Can you work these out from the model? Positions are in its coordinate system, mm. A direction names the side the tool comes from. Coordinates: 2 decimals unless noted, no trailing zeros. Order: outer loops, then holes, each group sorted by start corner. A loop starts at its lowest first (then second) coordinate and runs counter-clockwise, first axis right, second up. Notation, with made-up numbers: (44.25, -5) -> (103.25, -5) arc R30 ccw to (103.25, 19) -> close; hole circle Ø11 at (72.5, -6). An arc over 180 degrees is marked (long way). Answer as a JSON object with one key per item and string values. Group by question number.
(1) I want a section at D-D, the plane x = -5.25. List the corners of the cut face in (y, z) for me (3 decimals).
(2) I want a section at A-A, the plane x = 0. List the corners of the cut face in (y, z) for me (3 decimals).
(3) I want a section at B-B, the plane z = 3. List the corners of the cut face in (x, y) for me.
(4) For pin 1 (2 mm diameter, centred on y = -1, z = 18.5, fed in from +X); pin 2 (4.5 mm diameter, centred on x = -2.5, z = 14.5, fed in from +Y); pin 3 (0.8 mm diameter, centred on y = 0, z = -33, fed in from +X) (3 decimals), each with a flat end and sliding along its axis, tell me the tip position at first contact or that it passes through.
(5) I need wall thicknesses on line 1 (Z direction, x = -8.5, y = -2); line 2 (Y direction, x = -8, z = 7.5); line 3 (Z direction, x = -13, y = -12). Which ranges of each line are inside material? Lowest first, please.
(6) Which directions (+Z, -Z, +X, -X, +Y, -Y) give clear straight access to the entire face, cutting with the end or side of a thin tool? Please do faces 1 (the flat face through (-12, 12, 0)), 2 (the flat face through (9, 0.375, -33)), 3 (the cylindrical face through (15.62, 4.92, -15.16)), 4 (the flat face through (-9, -0.375, -33)), 5 (the cylindrical face through (1.096, -2.107, 31.836)).
(7) I want a section at C-C, the plane y = -8.5. List the corners of the cut face in (x, z) for me, plus the area to 3 significant figures.
from build123d import *

# Parameters (mm, degrees)
PAD_DEPTH    = 27.3
SKETCH001_R  = 16.375
PAD001_DEPTH = 30.75
SKETCH002_R  = 2.375
PAD002_DEPTH = 36.5
SKETCH004_W  = 2
SKETCH004_H  = 0.75
PAD004_DEPTH = 35


with BuildPart() as part:
    # Sketch → Pad (new body)
    with BuildSketch(Plane.XY):
        with BuildLine():
            Line((-16.25, 7.500021), (-16.25, -7.5))
            ThreePointArc((-16.25, -7.5), (-13.687184, -13.687185), (-7.499999, -16.25))
            Line((-7.499999, -16.25), (7.500022, -16.25))
            ThreePointArc((7.500022, -16.25), (13.687191, -13.687191), (16.25, -7.500023))
            Line((16.25, -7.500023), (16.25, 7.499999))
            ThreePointArc((16.25, 7.499999), (13.687185, 13.687184), (7.5, 16.25))
            Line((7.5, 16.25), (-7.500021, 16.25))
            ThreePointArc((-7.500021, 16.25), (-13.687184, 13.687184), (-16.25, 7.500021))
        make_face()
    extrude(amount=PAD_DEPTH)

    # Sketch001 → Pad001 (join)
    with BuildSketch(Plane.XY):
        Circle(SKETCH001_R)
    extrude(amount=-PAD001_DEPTH)

    # Sketch002 → Pad002 (join)
    with BuildSketch(Plane.XY):
        Circle(SKETCH002_R)
        with Locations((-5.25, 12.25)):
            Circle(SKETCH002_R)
    extrude(amount=PAD002_DEPTH)

    # Sketch004 → Pad004 (join)
    with BuildSketch(Plane.XY):
        with Locations((-8.875, 0)):
            Rectangle(SKETCH004_W, SKETCH004_H)
        with Locations((8.875, 0)):
            Rectangle(SKETCH004_W, SKETCH004_H)
    extrude(amount=-PAD004_DEPTH)


solid = part.part
Computed values:
{
 "1": {"outline": "(-16.25, 0) -> (-15.511, 0) -> (-15.511, -30.75) -> (15.511, -30.75) -> (15.511, 0) -> (16.25, 0) -> (16.25, 27.3) -> (14.625, 27.3) -> (14.625, 36.5) -> (9.875, 36.5) -> (9.875, 27.3) -> (-16.25, 27.3) -> close"},
 "2": {"outline": "(-16.375, -30.75) -> (16.375, -30.75) -> (16.375, 0) -> (16.25, 0) -> (16.25, 27.3) -> (2.375, 27.3) -> (2.375, 36.5) -> (-2.375, 36.5) -> (-2.375, 27.3) -> (-16.25, 27.3) -> (-16.25, 0) -> (-16.375, 0) -> close"},
 "3": {"outline": "(-16.25, -7.5) arc R8.75 ccw to (-7.5, -16.25) -> (7.5, -16.25) arc R8.75 ccw to (16.25, -7.5) -> (16.25, 7.5) arc R8.75 ccw to (7.5, 16.25) -> (-7.5, 16.25) arc R8.75 ccw to (-16.25, 7.5) -> close"},
 "4": {"pin 1": "stops at x = 16.25", "pin 2": "stops at y = 16.25", "pin 3": "stops at x = 9.875"},
 "5": {"line 1": "z = -30.75 to 27.3", "line 2": "y = -16.24 to 16.24", "line 3": "z = 0 to 27.3"},
 "6": {"face 1": "-Z, -X, +Y", "face 2": "-Z, +X, -X, +Y", "face 3": "-Z", "face 4": "-Z, +X, -X, -Y", "face 5": "+Z"},
 "7": {"outline": "(-16.19, 0) -> (-14, 0) -> (-14, -30.75) -> (14, -30.75) -> (14, 0) -> (16.19, 0) -> (16.19, 27.3) -> (-16.19, 27.3) -> close", "area": "1,740 mm2"}
}
